Autodesk Inventor part; units mm, degrees
ref_plane "YZ Plane" through (0, 0, 0) normal (1, 0, 0) x (0, 1, 0)
ref_plane "XZ Plane" through (0, 0, 0) normal (0, 1, 0) x (-1, 0, 0)
ref_plane "XY Plane" through (0, 0, 0) normal (0, 0, 1) x (1, 0, 0)
sketch "Sketch1" plane through (0, 0, 0) normal (0, 0, 1) x (1, 0, 0)
  line L0 (43.4638, 27.4592) -> (30.7638, 27.4592)
  line L1 (30.7638, 27.4592) -> (30.7638, 14.7592)
  line L2 (43.4638, 14.7592) -> (43.4638, 27.4592)
  line L3 (30.7638, 14.7592) -> (11.7138, 14.7592)
  line L4 (11.7138, 14.7592) -> (11.7138, 2.0592)
  line L5 (11.7138, 2.0592) -> (43.4638, 2.0592)
  line L6 (43.4638, 2.0592) -> (43.4638, 14.7592)
  point P0 (0, 0)
  dimension "d1" = 12.7
  dimension "d2" = 31.75
  dimension "d3" = 12.7
extrude "Extrusion1" add sketch "Sketch1" along normal blind 19.05
fillet "Fillet1" radius 6.35 2 edges at (11.7138, 8.4092, 19.05) (11.7138, 8.4092, 0)
sketch "Sketch2" plane through (30.7638, 14.7592, 19.05) normal (0, 1, 0) x (1, 0, 0)
  circle A0 centre (-9.525, 9.525) radius 4.7625
  point P0 (-30.7638, 19.05)
  point P1 (-31.0867, 15.9672)
  dimension "d8" = 9.525
hole "Hole1" at (21.2388, 14.7592, 9.525) at (-0.3229, 14.7592, 3.0828) at (21.2388, 14.7592, 9.525) direction (0, -1, 0) diameter 9.525 depth 25.4 tip angle 118
sketch "Sketch4" plane through (0, 0, 19.05) normal (0, 0, 1) x (1, 0, 0)
  line L0 (75.2138, 14.7592) -> (75.2138, 2.0592)
  line L1 (75.2138, 2.0592) -> (43.4638, 2.0592)
  line L2 (43.4638, 2.0592) -> (43.4638, 27.4592)
  line L3 (43.4638, 27.4592) -> (56.1638, 27.4592)
  line L4 (56.1638, 27.4592) -> (56.1638, 14.7592)
  line L5 (56.1638, 14.7592) -> (75.2138, 14.7592)
  point P0 (0, 0)
  dimension "d16" = 31.75
  dimension "d17" = 12.7
extrude "Extrusion3" add sketch "Sketch4" against normal blind 19.05
sketch "Sketch6" plane through (56.1638, 14.7592, 19.05) normal (0, 1, 0) x (1, 0, 0)
  line L0 (-38.1, 19.05) -> (19.05, 19.05)
  point P0 (-56.1638, 19.05)
  point P1 (9.525, 9.525)
hole "Hole2" at (65.6888, 14.7592, 9.525) direction (0, -1, 0) diameter 9.525 end through all
fillet "Fillet4" radius 2.54 1 edges at (30.7638, 14.7592, 9.525)
fillet "Fillet5" radius 2.54 1 edges at (56.1638, 14.7592, 9.525)
properties part number "Mirror"
Work out the finished part from the listing and answer in its coordinate system (mm). A direction names the side the tool comes from. Give positions to 0.01 mm unless a question says otherwise; leave off trailing zeros. Loops run counter-clockwise (first coordinate to the right, second up) from the corner with the lowest first, then second, coordinate; pieces in that order, holes last. Notation, with made-up numbers: (43, 59.5) -> (75, 59.5) arc R11 cw to (75, 72.5) -> close; hole circle Ø1 at (-3, 17). An arc over 180 degrees is marked (long way). Put each result on its own line as item: value. Start each with the question number.
Item 1: The part is cut by section D-D (z = 17.25). Give the vertices of the cut face in (x, y), then the cut area to 3 significant figures.
Item 2: The part is cut by section A-A (x = 67). Give the vertices of the cut face in (y, z).
Item 3: Each of these flat-tipped pins is pushed along its axis until it touches: P1, Ø8.5, axis at x = 19.5, z = 11.5, coming from the +Y side; P2, Ø3, axis at x = 56.5, z = 14.5, coming from the +Y side; P3, Ø3, axis at y = 20.5, z = 16.5, coming from the +X side; P4, Ø11, axis at y = 21, z = 14, coming from the -X side. Where does it stop, or does it pass through?
Item 4: The part is cut by section C-C (z = 11). Give the vertices of the cut face in (x, y), then the cut area to 3 significant figures.
Item 5: Find the intervals of material crossed by L1, parallel to X at y = 11.75, z = 9.5; L2, parallel to Y at x = 61, z = 18.5, in increasing order. Write a range as [from, to].
Item 6: Which of the six approach directions +Z, -Z, +X, -X, +Y, -Y give full straight-line access (tool end or side, diameter ignored) to faces 4 (the face through (30.764, 22, 9)), 5 (the face through (56.164, 22, 10)), 6 (the face through (43, 27.459, 10))?
Item 7: The part is cut by section B-B (y = 11). State how many separate pieces and enclosed holes the cut face has, then the cut area to 3 significant figures.
Item 8: The mould has two halves that part along Z. Classify faces 1 (the face through (62.47, 8.32, 6.015)), 2 (the face through (71, 14.759, 10)), 3 (the face through (13.623, 8.32, 17.239)): released by +Z, released by -Z, zero draft, split by the parting line, or undercut.
Answers below:
1. outline: (13.63, 2.06) -> (75.21, 2.06) -> (75.21, 14.76) -> (58.7, 14.76) arc R2.54 cw to (56.16, 17.3) -> (56.16, 27.46) -> (30.76, 27.46) -> (30.76, 17.3) arc R2.54 cw to (28.22, 14.76) -> (13.63, 14.76) -> close
1. area: 1,110 mm2
2. outline: (2.06, 0) -> (14.76, 0) -> (14.76, 4.95) -> (2.06, 4.95) -> close; (2.06, 14.1) -> (14.76, 14.1) -> (14.76, 19.05) -> (2.06, 19.05) -> close
3. P1: y = 14.76
3. P2: y = 27.46
3. P3: x = 56.16
3. P4: x = 30.02
4. outline: (11.71, 2.06) -> (16.71, 2.06) -> (16.71, 14.76) -> (11.71, 14.76) -> close; (25.77, 2.06) -> (61.16, 2.06) -> (61.16, 14.76) -> (58.7, 14.76) arc R2.54 cw to (56.16, 17.3) -> (56.16, 27.46) -> (30.76, 27.46) -> (30.76, 17.3) arc R2.54 cw to (28.22, 14.76) -> (25.77, 14.76) -> close; (70.22, 2.06) -> (75.21, 2.06) -> (75.21, 14.76) -> (70.22, 14.76) -> close
4. area: 902 mm2
5. L1: [11.71, 16.48], [26, 60.93], [70.45, 75.21]
5. L2: [2.06, 14.76]
6. face 4: +Z, -Z, -X, +Y
6. face 5: +Z, -Z, +X, +Y
6. face 6: +Z, -Z, +X, -X, +Y
7. separate pieces: 1
7. enclosed holes: 2
7. area: 1,050 mm2
8. face 1: undercut
8. face 2: zero draft
8. face 3: released by +Z
